Input: dimensioned drawing with shaded views. Units: mm. Origin: part minimum x, y, z. A direction names the side the tool comes from. Round coordinates to 2 decimals unless told otherwise and drop trailing zeros. Order: outer loops, then holes, each group sorted by start corner. A loop starts at its lowest first (then second) coordinate and runs counter-clockwise, first axis right, second up.
Item 1: Cut plane B-B on y = 279. Output: boundary loops of the cut face in (x, z).
Item 2: Reachability of the marked faces 1 and 2 from +Z, -Z, +X, -X, +Y, -Y: full face, straight path, thin tool, end or side. Return the list, or none.
Item 3: First-contact query: pin 1 (1 mm diameter, centred on x = 413.5, z = 419.5, fed in from +Y). Flat tip, straight axial feed; report the tip coordinate or a pass-through.
Item 4: Mould query, pull axis Z, two halves, no side actions, for the marked faces 3, 4 and 5. Classes: released by +Z, released by -Z, zero draft, split by the parting line, or undercut.
Item 5: Line query: L1, parallel to X at y = 528.5, z = 441; L2, parallel to Z at x = 238.5, y = 82.5; L3, parallel to Y at x = 285.5, z = 166. Output: solid intervals per line, ascending.
Item 6: Cut plane C-C on x = 239.5. Output: boundary loops of the cut face in (y, z), then the cut area to 3 significant figures.
Item 7: Cut plane A-A on z = 558. Output: boundary loops of the cut face in (x, y), then the cut area to 3 significant figures.
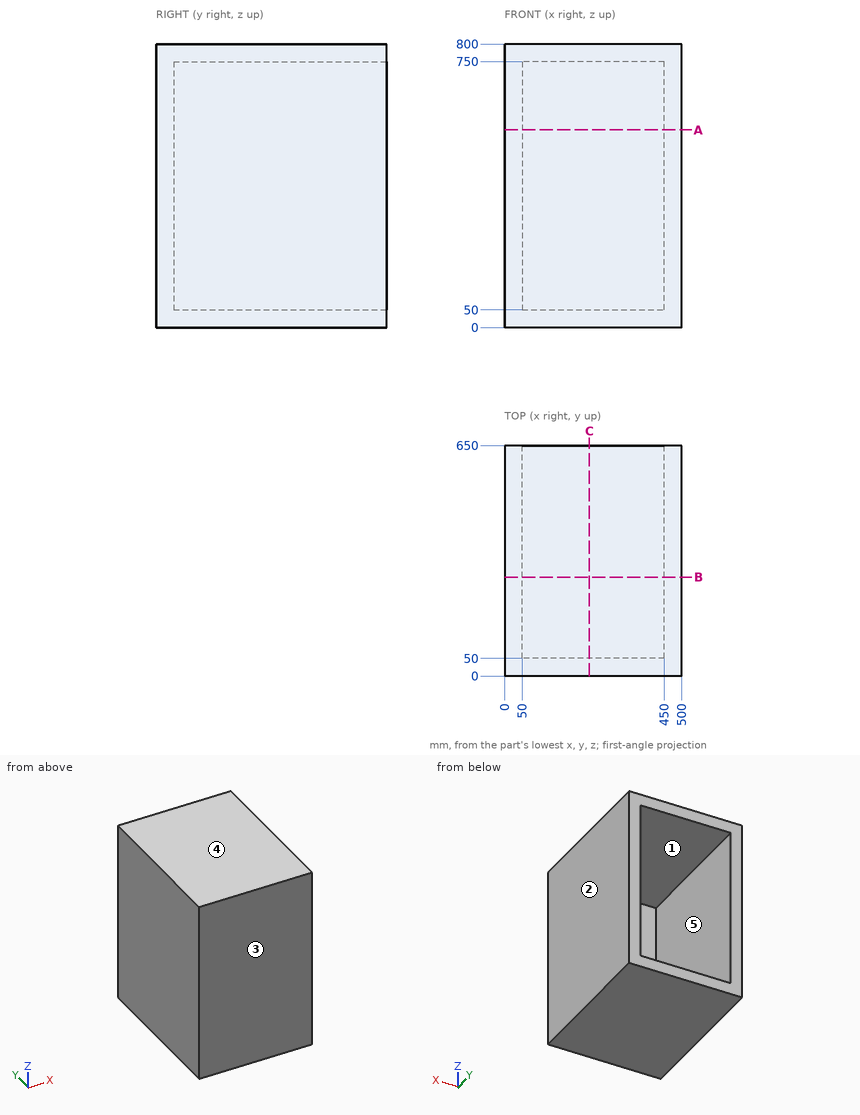
From the geometry:
1. outline: (0, 0) - (500, 0) - (500, 800) - (0, 800) - close; hole (50, 50) - (450, 50) - (450, 750) - (50, 750) - close
2. face 1: +Y
2. face 2: +Z, -Z, +X, +Y, -Y
3. pin 1: stops at y = 50
4. face 3: zero draft
4. face 4: released by +Z
4. face 5: undercut
5. L1: x = 0 to 50, 450 to 500
5. L2: z = 0 to 50, 750 to 800
5. L3: y = 0 to 50
6. outline: (0, 0) - (650, 0) - (650, 50) - (50, 50) - (50, 750) - (650, 750) - (650, 800) - (0, 800) - close
6. area: 100,000 mm2
7. outline: (0, 0) - (500, 0) - (500, 650) - (450, 650) - (450, 50) - (50, 50) - (50, 650) - (0, 650) - close
7. area: 85,000 mm2
